Geometry: final body of the model. Coordinates: model frame, mm. A direction names the side the tool comes from. Round coordinates to 2 decimals unless told otherwise and drop trailing zeros. Order: outer loops, then holes, each group sorted by start corner. A loop starts at its lowest first (then second) coordinate and runs counter-clockwise, first axis right, second up. Notation, with made-up numbers: M -7,-3.5 L 44,-3.5 A30 cw 44,33.5 Z; hole C 9.25,-21 d3. An arc over 180 degrees is marked long. Return JSON: item names as keys, results as strings. Group by question number.
Q1. Cut plane B-B on x = 0. Output: boundary loops of the cut face in (y, z) (3 decimals).
Q2. Mould query, pull axis Z, two halves, no side actions, for faces 3 (the face through (4.72, -13.38, -9.07)), 4 (the face through (38.158, -112.7, 12.016)), 5 (the face through (6, -228.6, 30)). Classes: released by +Z, released by -Z, zero draft, split by the parting line, or undercut.
Q3. Ray query, probe 1 along X at (y, z) = (-90, 1); probe 2 along Z at (x, y) = (0, -5) (3 decimals); probe 3 along Z at (x, y) = (0, -110) (3 decimals). Return the intervals inside material, ascending.
Q4. Cut plane A-A on z = 0. Output: boundary loops of the cut face in (x, y) (3 decimals), and give its area (3 significant figures).
Q5. Contact query for flat-ended pins moving along their axis: pin 1 (6 mm diameter, centred on x = -22, z = 24, fed in from +Y); pin 2 (1.5 mm diameter, centred on x = 29, z = -5, fed in from -Y); pin 3 (2 mm diameter, centred on y = -108, z = 14.5, fed in from +X); pin 4 (5 mm diameter, centred on y = -96, z = -16, fed in from -X). Output: stop coordinate, or through.
Q6. Cut plane C-C on y = -179. Output: boundary loops of the cut face in (x, z) (3 decimals), and give its area (3 significant figures).
Q7. Access query for faces 1 (the face through (22.278, -125.578, 20.428)), 2 (the face through (-9, 0, 1)). Directions: +Z, -Z, +X, -X, +Y, -Y. A direction counts if a zero-diameter tool reaches every point of the face in a straight line with its end or side. Return the directions, or none.
Q8. Cut plane D-D on x = 35. Output: boundary loops of the cut face in (y, z), and give its area (3 significant figures).
```python
from build123d import *

# Parameters (mm, degrees)
F0_R     = 40.005
F1_DEPTH = 228.6
F3_D     = 60.452
F3_DEPTH = 203.2
F3_TIP   = 18.1616130707
F5_D     = 17.78


with BuildPart() as f1:
    # F0 (on Front) → F1 (new body)
    with BuildSketch(Plane.XZ):
        Circle(F0_R)
    extrude(amount=F1_DEPTH)

    # F3
    with Locations(Plane.XZ.offset(228.6)):
        with Locations((0, 0)):
            Hole(F3_D / 2, depth=F3_DEPTH)
            with Locations((0, 0, -(F3_DEPTH + F3_TIP / 2))):  # 118° drill point
                Cone(0, F3_D / 2, F3_TIP, mode=Mode.SUBTRACT)

    # F5 (through all)
    with Locations(Plane(origin=(0, 0, 0), x_dir=(-1, 0, 0), z_dir=(0, 1, 0))):
        with Locations((0, 0)):
            Hole(F5_D / 2)


solid = f1.part
```
Result sheet:
{
 "1": {"outline": "M -228.6,-40.005 L 0,-40.005 L 0,-8.89 L -12.58,-8.89 L -25.4,-30.226 L -228.6,-30.226 Z; M -228.6,30.226 L -25.4,30.226 L -12.58,8.89 L 0,8.89 L 0,40.005 L -228.6,40.005 Z"},
 "2": {"face 3": "undercut", "face 4": "split by the parting line", "face 5": "zero draft"},
 "3": {"probe 1": "x = -39.99 to -30.21, 30.21 to 39.99", "probe 2": "z = -40.005 to -8.89, 8.89 to 40.005", "probe 3": "z = -40.005 to -30.226, 30.226 to 40.005"},
 "4": {"outline": "M -40.005,-228.6 L -30.226,-228.6 L -30.226,-25.4 L -8.89,-12.58 L -8.89,0 L -40.005,0 Z; M 8.89,-12.58 L 30.226,-25.4 L 30.226,-228.6 L 40.005,-228.6 L 40.005,0 L 8.89,0 Z", "area": "5,280 mm²"},
 "5": {"pin 1": "stops at y = 0", "pin 2": "stops at y = -25.37", "pin 3": "stops at x = 37.66", "pin 4": "stops at x = -37.66"},
 "6": {"outline": "C 0,0 d80.01; hole C 0,0 d60.452", "area": "2,160 mm²"},
 "7": {"face 1": "-Y", "face 2": "+Z, -Z, +X, -X, +Y"},
 "8": {"outline": "M -228.6,-19.38 L 0,-19.38 L 0,19.38 L -228.6,19.38 Z", "area": "8,860 mm²"}
}
